Design review of the part built by this model. Coordinates are the model's own, in mm. A direction names the side the tool comes from. Coordinates: 2 decimals unless noted, no trailing zeros. Loops run counter-clockwise (first coordinate to the right, second up) from the corner with the lowest first, then second, coordinate; pieces in that order, holes last. Notation, with made-up numbers: (81.25, 3) - (130.25, 3) arc R37 ccw to (130.25, 42) - close; hole circle Ø4 at (79.5, 45.25). An arc over 180 degrees is marked (long way). Return JSON: item names as keys, results as strings. Group by question number.
from build123d import *

# Parameters (mm, degrees)
BOSS_EXTRUDE1_DEPTH  = 4
FILLET1_R            = 9.5
M3_CLEARANCE_HOLE1_D = 3.2
M5_CLEARANCE_HOLE1_D = 5.3
FILLET2_R            = 0.2


with BuildPart() as part:
    # Sketch1 → Boss-Extrude1 (new body)
    with BuildSketch(Plane.XY):
        Polygon((73.262039089, -348.953453607), (106.008421642, -348.953453607), (106.008421642, -312.503453607), (125.368421642, -312.503453607), (125.368421642, -277.953453607), (107.148421642, -277.953453607), (107.148421642, -302.953453607), (73.262039089, -302.953453607), align=None)
    extrude(amount=-BOSS_EXTRUDE1_DEPTH)

    # Fillet1
    fillet1_edges = [part.edges().sort_by_distance(p)[0] for p in [
        (73.262039089, -302.953453607, -2),
        (107.148421642, -302.953453607, -2),
        (125.368421642, -312.503453607, -2),
        (106.008421642, -312.503453607, -2),
        (106.008421642, -348.953453607, -2),
        (73.262039089, -348.953453607, -2),
    ]]
    fillet(fillet1_edges, radius=FILLET1_R)

    # M3 Clearance Hole1 (through all)
    with Locations(Plane.XY):
        with Locations((116.258421642, -290.703453607), (91.348421642, -319.203453607)):
            Hole(M3_CLEARANCE_HOLE1_D / 2)

    # M5 Clearance Hole1 (through all)
    with Locations(Plane.XY):
        with Locations((79.612142542, -343.223274497)):
            Hole(M5_CLEARANCE_HOLE1_D / 2)

    # Fillet2
    fillet2_edges = [part.edges().sort_by_distance(p)[0] for p in [
        (107.148421642, -277.953453607, -2),
        (125.368421642, -277.953453607, -2),
    ]]
    fillet(fillet2_edges, radius=FILLET2_R)


solid = part.part
Item 1: For P1, Ø8, axis at x = 116, y = -297, coming from the +Z side; P2, Ø2, axis at y = -323.5, z = -2, coming from the +X side, all flat-tipped, find the tip position at first contact; note any pin that passes through.
Item 2: Add section B-B (x = 85.5). State the section outline as (y, z) points, then the cut area to 3 significant figures.
Item 3: Add section A-A (z = -1.5). State the section outline as (x, y) points, then the cut area to 3 significant figures.
Item 4: To check wall thickness, follow line 1 (X direction, y = -289, z = -2.4); line 2 (X direction, y = -291, z = -1.45); line 3 (X direction, y = -319.5, z = -0.4). State the ranges of each line that lie inside material, in increasing order. Write a range as from..to.
Item 5: Draft analysis for pull direction Y (two halves, no side actions). For faces 4 (the face through (116, -277.953, -2)), 5 (the face through (90, -348.953, -2)), 6 (the face through (80.19, -345.81, -2.03)), state which applies: pulls with the +Y half, pulls with the -Y half, needs draft (parallel to the pull), parting line crosses it, or undercut.
Item 6: For faces 1 (the face through (107.148, -286, -2)), 2 (the face through (106.008, -331, -2)), 3 (the face through (76.119, -346.244, -2.028)), list the 3-axis set-ups (+Z, -Z, +X, -X, +Y, -Y) from which the entire face can be reached by the end or side of a thin tool; tool diameter is ignored.
Item 7: Add section C-C (y = -327.5). State the section outline as (x, z) points.
Answers below:
{
 "1": {"P1": "stops at z = 0", "P2": "stops at x = 106.01"},
 "2": {"outline": "(-348.95, -4) - (-302.95, -4) - (-302.95, 0) - (-348.95, 0) - close", "area": "184 mm^2"},
 "3": {"outline": "(73.26, -339.45) arc R9.5 ccw to (82.76, -348.95) - (96.51, -348.95) arc R9.5 ccw to (106.01, -339.45) - (106.01, -322) arc R9.5 cw to (115.51, -312.5) - (115.87, -312.5) arc R9.5 ccw to (125.37, -303) - (125.37, -278.15) arc R0.2 ccw to (125.17, -277.95) - (107.35, -277.95) arc R0.2 ccw to (107.15, -278.15) - (107.15, -293.45) arc R9.5 cw to (97.65, -302.95) - (82.76, -302.95) arc R9.5 ccw to (73.26, -312.45) - close; hole circle Ø5.3 at (79.61, -343.22); hole circle Ø3.2 at (91.35, -319.2); hole circle Ø3.2 at (116.26, -290.7)", "area": "2,070 mm^2"},
 "4": {"line 1": "x = 107.15..125.37", "line 2": "x = 107.15..114.69, 117.83..125.37", "line 3": "x = 73.26..89.78, 92.92..106.34"},
 "5": {"face 4": "pulls with the +Y half", "face 5": "pulls with the -Y half", "face 6": "undercut"},
 "6": {"face 1": "+Z, -Z, -X, +Y", "face 2": "+Z, -Z, +X, -Y", "face 3": "+Z, -Z, -X, -Y"},
 "7": {"outline": "(73.26, -4) - (106.01, -4) - (106.01, 0) - (73.26, 0) - close"}
}
